Geometry check sheet. Reference: the model listing, model coordinates, mm. A direction names the side the tool comes from. Round coordinates to 2 decimals unless told otherwise and drop trailing zeros. Loops run counter-clockwise (first coordinate to the right, second up) from the corner with the lowest first, then second, coordinate; pieces in that order, holes last. Notation, with made-up numbers: M 43,-0.5 L 87,-0.5 A7 ccw 87,7.5 Z; hole C 12,-18 d5. An arc over 180 degrees is marked long. Use one line per item in the form item = value. Start each with the question number.
1. Material ranges on line 1 (Y direction, x = 0, z = 2.9); line 2 (Z direction, x = -1.05, y = 1.35); line 3 (X direction, y = -0.15, z = 2.25), recorded low to high.
2. Cross-section at D-D (z = -2.5). Record the boundary of the cut face in (x, y).
3. Draft check along X on faces 1 (the flat face through (2.026, -1.191, 2.465)), 2 (the flat face through (0, 0, -6)), 3 (the flat face through (0, 0, 0)). Enter one of: pulls with the +X half, pulls with the -X half, needs draft (parallel to the pull), parting line crosses it, or undercut.
4. Cross-section at B-B (x = 0). Record the boundary of the cut face in (y, z), then the cut area to 3 significant figures.
5. Set-up check for faces 4 (the cylindrical face through (-0.27, 1.22, -2.96)), 5 (the flat face through (0, -2.35, 2)), 6 (the cylindrical face through (0, -1, 2)): record each of +Z, -Z, +X, -X, +Y, -Y from which the full face is reachable in a straight line by a thin tool's end or side.
6. Cross-section at A-A (z = 4). Record the boundary of the cut face in (x, y).
7. Go/stop test with flat-tipped pins: pin 1 (1 mm diameter, centred on x = -0.5, z = -2.5, fed in from +Y); pin 2 (0.6 mm diameter, centred on x = 0, y = 0, fed in from +Z); pin 3 (2 mm diameter, centred on x = 0.5, z = -2, fed in from -Y). Record where each tip stops, or that it passes through.
8. Cross-section at C-C (y = -0.2). Record the boundary of the cut face in (x, z), then the cut area to 3 significant figures.
```python
from build123d import *

# Parameters (mm, degrees)
SKETCH_R     = 1
PAD_DEPTH    = 5
SKETCH001_R  = 1.25
PAD001_DEPTH = 6


with BuildPart() as part:
    # Sketch → Pad (new body)
    with BuildSketch(Plane.XY):
        Polygon((1.356773, -2.35), (2.713546, 0), (1.356773, 2.35), (-1.356773, 2.35), (-2.713546, 0), (-1.356773, -2.35), align=None)
        Circle(SKETCH_R, mode=Mode.SUBTRACT)
    extrude(amount=PAD_DEPTH)

    # Sketch001 (on Face8 of Pad) → Pad001 (join)
    with BuildSketch(Plane(origin=(0, 0, 0), x_dir=(1, 0, 0), z_dir=(0, 0, -1))):
        Circle(SKETCH001_R)
    extrude(amount=PAD001_DEPTH)


solid = part.part
```
Reported:
q1.line_1 = -2.35 to -1, 1 to 2.35
q1.line_2 = 0 to 5
q1.line_3 = -2.63 to -0.99, 0.99 to 2.63
q2.outline = C 0,0 d2.5
q3.face_1 = pulls with the +X half
q3.face_2 = needs draft
q3.face_3 = undercut
q4.outline = M -2.35,0 L -1.25,0 L -1.25,-6 L 1.25,-6 L 1.25,0 L 2.35,0 L 2.35,5 L 1,5 L 1,0 L -1,0 L -1,5 L -2.35,5 Z
q4.area = 28.5 mm²
q5.face_4 = -Z
q5.face_5 = +Z, -Z, +X, -X, -Y
q5.face_6 = +Z
q6.outline = M -2.71,0 L -1.36,-2.35 L 1.36,-2.35 L 2.71,0 L 1.36,2.35 L -1.36,2.35 Z; hole C 0,0 d2
q7.pin_1 = 1.25
q7.pin_2 = 0
q7.pin_3 = -1.25
q8.outline = M -2.6,0 L -1.23,0 L -1.23,-6 L 1.23,-6 L 1.23,0 L 2.6,0 L 2.6,5 L 0.98,5 L 0.98,0 L -0.98,0 L -0.98,5 L -2.6,5 Z
q8.area = 31.0 mm²
